Part model, mm, in its own coordinate system. A direction names the side the tool comes from. Round coordinates to 2 decimals unless told otherwise and drop trailing zeros. Loops run counter-clockwise (first coordinate to the right, second up) from the corner with the lowest first, then second, coordinate; pieces in that order, holes last. Notation, with made-up numbers: (65, 40) -> (113, 40) arc R27 ccw to (113, 62) -> close; hole circle Ø6 at (65.5, -8). An arc over 180 degrees is marked (long way). Answer as CSV lines item,"result".
from build123d import *

# Parameters (mm, degrees)
ESQUISSE1_W        = 66
ESQUISSE1_H        = 29.5
BOSS_EXTRU_1_DEPTH = 57
ESQUISSE2_R        = 9
BOSS_EXTRU_2_DEPTH = 2
ESQUISSE3_R        = 4
BOSS_EXTRU_3_DEPTH = 6
BOSS_EXTRU_4_START = 40
ESQUISSE4_W        = 82
ESQUISSE4_H        = 29.5
ESQUISSE4_R        = 1.5
BOSS_EXTRU_4_DEPTH = 7
ESQUISSE5_W        = 7
ESQUISSE5_H        = 4
BOSS_EXTRU_5_DEPTH = 6


with BuildPart() as part:
    # Esquisse1 → Boss.-Extru.1 (new body)
    with BuildSketch(Plane(origin=(0, 0, 0), x_dir=(1, 0, 0), z_dir=(0, 1, 0))):
        with Locations((-19, 0)):
            Rectangle(ESQUISSE1_W, ESQUISSE1_H)
    extrude(amount=BOSS_EXTRU_1_DEPTH)

    # Esquisse2 → Boss.-Extru.2 (add)
    with BuildSketch(Plane(origin=(0, 57, 0), x_dir=(1, 0, 0), z_dir=(0, 1, 0))):
        with Locations(Location((0, 0, 0), (0, 0, 270))):
            Circle(ESQUISSE2_R)
    extrude(amount=BOSS_EXTRU_2_DEPTH)

    # Esquisse3 → Boss.-Extru.3 (add)
    with BuildSketch(Plane(origin=(0, 59, 0), x_dir=(1, 0, 0), z_dir=(0, 1, 0))):
        with Locations(Location((0, 0, 0), (0, 0, 270))):
            Circle(ESQUISSE3_R)
    extrude(amount=BOSS_EXTRU_3_DEPTH)

    # Esquisse4 → Boss.-Extru.4 (add)
    with BuildSketch(Plane(origin=(0, 0, 0), x_dir=(1, 0, 0), z_dir=(0, 1, 0)).offset(BOSS_EXTRU_4_START)):
        with Locations((-19, 0)):
            Rectangle(ESQUISSE4_W, ESQUISSE4_H)
        with Locations(Location((-56, 9, 0), (0, 0, 270))):
            Circle(ESQUISSE4_R, mode=Mode.SUBTRACT)
        with Locations(Location((-56, -9, 0), (0, 0, 90))):
            Circle(ESQUISSE4_R, mode=Mode.SUBTRACT)
        with Locations(Location((18, -9, 0), (0, 0, 270))):
            Circle(ESQUISSE4_R, mode=Mode.SUBTRACT)
        with Locations(Location((18, 9, 0), (0, 0, 90))):
            Circle(ESQUISSE4_R, mode=Mode.SUBTRACT)
    extrude(amount=BOSS_EXTRU_4_DEPTH)

    # Esquisse5 → Boss.-Extru.5 (add)
    with BuildSketch(Plane(origin=(14, 0, 0), x_dir=(0, 0, -1), z_dir=(1, 0, 0))):
        with Locations((0, 5)):
            Rectangle(ESQUISSE5_W, ESQUISSE5_H)
    extrude(amount=BOSS_EXTRU_5_DEPTH)


solid = part.part
Q1. Drill centre lines: line 1 along X through (y, z) = (42, 9); line 2 along Y through (x, z) = (1.5, 5.5); line 3 along Y through (x, z) = (-36.5, -2.5). Where is each one in solid material? Low to high.
Geometry results:
line 1,"-60 to -57.5, -54.5 to 16.5, 19.5 to 22"
line 2,"0 to 59"
line 3,"0 to 57"
Q2. Saw through at C-C, the plane y = 4.5. Write the cut outline in (x, z), then the cut area to 3 significant figures.
Geometry results:
outline,"(-52, -14.75) -> (14, -14.75) -> (14, -3.5) -> (20, -3.5) -> (20, 3.5) -> (14, 3.5) -> (14, 14.75) -> (-52, 14.75) -> close"
area,"1,990 mm2"
Q3. Saw through at D-D, the plane z = -12. Write the cut outline in (x, y).
Geometry results:
outline,"(-60, 40) -> (-52, 40) -> (-52, 0) -> (14, 0) -> (14, 40) -> (22, 40) -> (22, 47) -> (14, 47) -> (14, 57) -> (-52, 57) -> (-52, 47) -> (-60, 47) -> close"
Q4. Saw through at A-A, the plane x = -56. Write the cut outline in (y, z), then the cut area to 4 significant figures.
Geometry results:
outline,"(40, -14.75) -> (47, -14.75) -> (47, -10.5) -> (40, -10.5) -> close; (40, -7.5) -> (47, -7.5) -> (47, 7.5) -> (40, 7.5) -> close; (40, 10.5) -> (47, 10.5) -> (47, 14.75) -> (40, 14.75) -> close"
area,"164.5 mm2"
Q5. Saw through at B-B, the plane x = 18. Write the cut outline in (y, z), then the cut area to 4 significant figures.
Geometry results:
outline,"(3, -3.5) -> (7, -3.5) -> (7, 3.5) -> (3, 3.5) -> close; (40, -14.75) -> (47, -14.75) -> (47, -10.5) -> (40, -10.5) -> close; (40, -7.5) -> (47, -7.5) -> (47, 7.5) -> (40, 7.5) -> close; (40, 10.5) -> (47, 10.5) -> (47, 14.75) -> (40, 14.75) -> close"
area,"192.5 mm2"
Q6. Two-plate mould, pull along Z, no slides. Class faces 5 (the face through (17, 5, -3.5)), 6 (the face through (16.99, 43.45, -7.89)), 7 (the face through (-3.905, 61.958, -0.867)): pulls with the +Z half, pulls with the -Z half, needs draft (parallel to the pull), parting line crosses it, or undercut.
Geometry results:
face 5,"pulls with the -Z half"
face 6,"undercut"
face 7,"parting line crosses it"
Q7. Drop flat-ended pins along their axis: P1, Ø9, axis at x = -33.5, z = 1.5, coming from the +Y side; P2, Ø6.5, axis at x = 19, z = -2, coming from the -Y side; P3, Ø3, axis at x = 16.5, y = 4.5, coming from the +Z side; P4, Ø1.8, axis at x = 18, z = 9, coming from the -Y side. Give the stop position or say it passes through.
Geometry results:
P1,"y = 57"
P2,"y = 3"
P3,"z = 3.5"
P4,"through"
Q8. Which spindle directions (+Z, -Z, +X, -X, +Y, -Y) get a long thin tool onto all of the face, cutting with end or side? Do faces 1 (the face through (-56, 40, 0)), 2 (the face through (17, 3, 0)), 3 (the face through (17, 5, 3.5)), 4 (the face through (-2, 59, 4)). Say none if no direction does.
Geometry results:
face 1,"+Z, -Z, -X, -Y"
face 2,"+Z, -Z, +X, -Y"
face 3,"+Z, +X, -Y"
face 4,"+Y"
